Part print with two shaded views. Sizes in mm from the minimum x, y, z corner. Give positions to 0.01 mm unless a question says otherwise; leave off trailing zeros. Write each loop counter-clockwise with the first axis right and the second up, starting at its lowest first coordinate (ties: lowest second). Pieces come first, ordered by that corner, then holes. Notation, with made-up numbers: (-28.75, 67) -> (-10.75, 67) arc R12 cw to (-10.75, 77) -> close; hole circle Ø5 at (6.25, 89.5). An arc over 180 degrees is marked (long way). Write item = value, one per line. Start each with the question number.
Q1. Saw through at C-C, the plane x = 30.25. List the corners of the cut face in (y, z).
Q2. Drop a flat-ended pin along its axis: P1, Ø4, axis at x = 30.25, y = 18.35, coming from the -Z side. Give the stop position or say it passes through.
Q3. Saw through at A-A, the plane y = 18.35. List the corners of the cut face in (x, z).
Q4. Saw through at B-B, the plane x = 203.9. List the corners of the cut face in (y, z).
Q5. Wall check: line 1 (X direction, y = 18.35, z = 1.5); line 2 (Y direction, x = 12, z = 2.75); line 3 (Y direction, x = 30.25, z = 1.5). Give the ranges that are in metal, low to high.
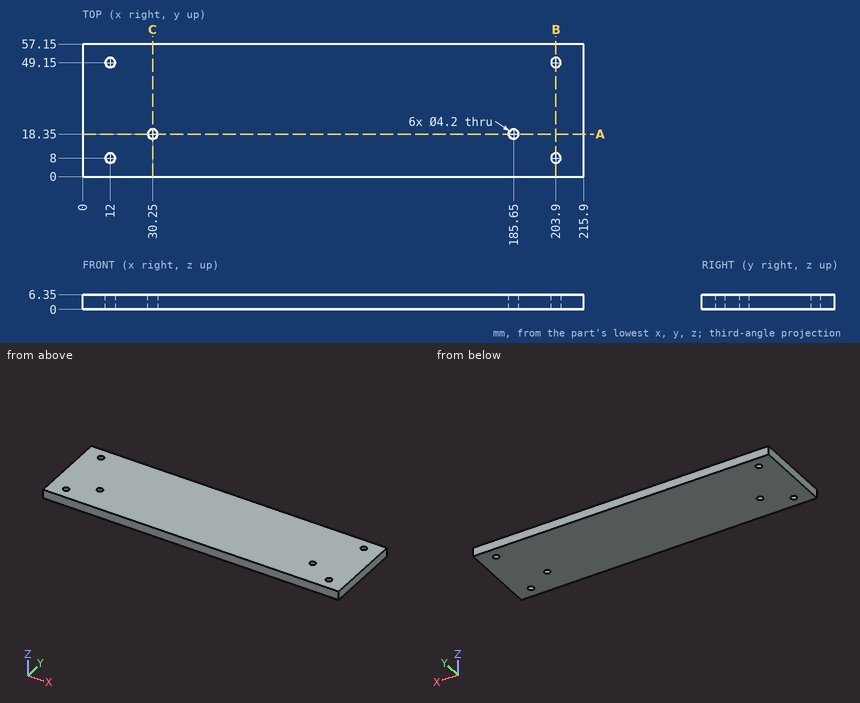
Report:
q1.outline = (0, 0) -> (16.25, 0) -> (16.25, 6.35) -> (0, 6.35) -> close; (20.45, 0) -> (57.15, 0) -> (57.15, 6.35) -> (20.45, 6.35) -> close
q2.P1 = through
q3.outline = (0, 0) -> (28.15, 0) -> (28.15, 6.35) -> (0, 6.35) -> close; (32.35, 0) -> (183.55, 0) -> (183.55, 6.35) -> (32.35, 6.35) -> close; (187.75, 0) -> (215.9, 0) -> (215.9, 6.35) -> (187.75, 6.35) -> close
q4.outline = (0, 0) -> (5.9, 0) -> (5.9, 6.35) -> (0, 6.35) -> close; (10.1, 0) -> (47.05, 0) -> (47.05, 6.35) -> (10.1, 6.35) -> close; (51.25, 0) -> (57.15, 0) -> (57.15, 6.35) -> (51.25, 6.35) -> close
q5.line_1 = 0 to 28.15, 32.35 to 183.55, 187.75 to 215.9
q5.line_2 = 0 to 5.9, 10.1 to 47.05, 51.25 to 57.15
q5.line_3 = 0 to 16.25, 20.45 to 57.15
